```python
from build123d import *

# Parameters (mm, degrees)
F0_W     = 95
F0_H     = 95
F1_DEPTH = 50
F2_R     = 12.7
F3_DEPTH = 10
F4_R     = 12.7
F5_DEPTH = 10


with BuildPart() as f1:
    # F0 (on Top) → F1 (new body)
    with BuildSketch(Plane.XY):
        Rectangle(F0_W, F0_H)
    extrude(amount=F1_DEPTH)

    # F2 (on face) → F3 (join)
    with BuildSketch(Plane.XZ.offset(47.5)):
        with Locations((12.5, 25)):
            Circle(F2_R)
    extrude(amount=F3_DEPTH)

    # F4 (on face) → F5 (join)
    with BuildSketch(Plane.YZ.offset(47.5)):
        with Locations((-12.5, 25)):
            Circle(F4_R)
    extrude(amount=F5_DEPTH)


solid = f1.part
```
Work out the finished part from the listing and answer in its coordinate system (mm). A direction names the side the tool comes from. Coordinates: 2 decimals unless noted, no trailing zeros. Order: outer loops, then holes, each group sorted by start corner. A loop starts at its lowest first (then second) coordinate and runs counter-clockwise, first axis right, second up. Notation, with made-up numbers: (-28, -8) - (6, -8) arc R29 cw to (6, 27) - close; hole circle Ø1 at (33.25, 59). An arc over 180 degrees is marked (long way). Answer as a JSON object with one key per item and string values.
1. Find section B-B on y = -12.5. Determine the outline of the cut face in (x, z).
Output values:
{"outline": "(-47.5, 0) - (47.5, 0) - (47.5, 12.3) - (57.5, 12.3) - (57.5, 37.7) - (47.5, 37.7) - (47.5, 50) - (-47.5, 50) - close"}
2. Find section A-A on z = 25. Determine the outline of the cut face in (x, y), plus the area to 3 significant figures.
Output values:
{"outline": "(-47.5, -47.5) - (-0.2, -47.5) - (-0.2, -57.5) - (25.2, -57.5) - (25.2, -47.5) - (47.5, -47.5) - (47.5, -25.2) - (57.5, -25.2) - (57.5, 0.2) - (47.5, 0.2) - (47.5, 47.5) - (-47.5, 47.5) - close", "area": "9,530 mm²"}
3. A tool of negligible diameter and unlimited length cuts with its end or side. For faces 1 (the face through (12, -57.5, 25)), 2 (the face through (52.43, -25.188, 25.558)), 3 (the face through (-0.188, -52.43, 25.558)), from which of +Z, -Z, +X, -X, +Y, -Y can it reach the whole face along a straight path? Write none if from no direction.
Output values:
{"face 1": "+Z, -Z, +X, -X, -Y", "face 2": "+X", "face 3": "-Y"}
4. Each of these flat-tipped pins is pushed along its axis until it touches: P1, Ø6, axis at y = -3.5, z = 39, coming from the +X side; P2, Ø1.5, axis at x = 44, z = 22.5, coming from the -Y side. Where does it stop, or does it pass through?
Output values:
{"P1": "stops at x = 47.5", "P2": "stops at y = -47.5"}
5. Find section D-D on y = 39. Determine the outline of the cut face in (x, z).
Output values:
{"outline": "(-47.5, 0) - (47.5, 0) - (47.5, 50) - (-47.5, 50) - close"}
6. Consider line 1 (X direction, y = -6.5, z = 13). Determine where the line is inside the solid, lowest interval first.
Output values:
{"line 1": "x = -47.5 to 47.5"}
7. Find section C-C on x = 12.5. Determine the outline of the cut face in (y, z).
Output values:
{"outline": "(-57.5, 12.3) - (-47.5, 12.3) - (-47.5, 0) - (47.5, 0) - (47.5, 50) - (-47.5, 50) - (-47.5, 37.7) - (-57.5, 37.7) - close"}
